Can you work these out from the model? Positions are in its coordinate system, mm. A direction names the side the tool comes from. Coordinates: 2 decimals unless noted, no trailing zeros. Order: outer loops, then holes, each group sorted by start corner. A loop starts at its lowest first (then second) coordinate and runs counter-clockwise, first axis right, second up. Notation, with made-up numbers: M -30,33 L 14,33 A14 ccw 14,44 Z; hole C 35.25,5.25 d8. An arc over 180 degrees is marked long. Answer as a JSON object with one key per item and string values.
from build123d import *

# Parameters (mm, degrees)
F1_DEPTH = 5.9944
F0_R     = 5.9944
F2_DEPTH = 13.0048
F0_R_2   = 13.0048
F3_DEPTH = 20.0025


with BuildPart() as f1:
    # F0 (on Front) → F1 (new body)
    with BuildSketch(Plane.XZ):
        with BuildLine():
            ThreePointArc((-12.0015, 0), (0, 12.0015), (12.0015, 0))
            ThreePointArc((12.0015, 0), (10.942664, -4.928905), (7.952988, -8.988102))
            Line((7.952988, -8.988102), (71.316989, 47.078591))
            ThreePointArc((71.316989, 47.078591), (78.103737, 50.03276), (85.331821, 48.438437))
            ThreePointArc((85.331821, 48.438437), (73.022425, 71.33485), (87.698507, 92.791308))
            Line((87.698507, 92.791308), (-4.940825, 50.942287))
            ThreePointArc((-4.940825, 50.942287), (6.509174, 50.087989), (12.0015, 40.005))
            ThreePointArc((12.0015, 40.005), (0, 28.0035), (-12.0015, 40.005))
            Line((-12.0015, 40.005), (-12.0015, 0))
        make_face()
    extrude(amount=F1_DEPTH)

    # F0 (on Front) → F2 (join)
    with BuildSketch(Plane.XZ):
        with BuildLine():
            ThreePointArc((-4.940825, 50.942287), (-10.082989, 46.514174), (-12.0015, 40.005))
            ThreePointArc((-12.0015, 40.005), (0, 28.0035), (12.0015, 40.005))
            ThreePointArc((12.0015, 40.005), (6.509174, 50.087989), (-4.940825, 50.942287))
        make_face()
        with Locations((0, 40.005)):
            Circle(F0_R, mode=Mode.SUBTRACT)
        with BuildLine():
            ThreePointArc((7.952988, -8.988102), (10.942664, -4.928905), (12.0015, 0))
            ThreePointArc((12.0015, 0), (0, 12.0015), (-12.0015, 0))
            ThreePointArc((-12.0015, 0), (-4.928905, -10.942664), (7.952988, -8.988102))
        make_face()
        Circle(F0_R, mode=Mode.SUBTRACT)
    extrude(amount=F2_DEPTH)

    # F0 (on Front) → F3 (join)
    with BuildSketch(Plane.XZ):
        with BuildLine():
            ThreePointArc((87.698507, 92.791308), (73.022425, 71.33485), (85.331821, 48.438437))
            ThreePointArc((85.331821, 48.438437), (110.416984, 48.30068), (122.9995, 70.0024))
            ThreePointArc((122.9995, 70.0024), (111.555701, 91.011294), (87.698507, 92.791308))
        make_face()
        with Locations((97.9932, 70.0024)):
            Circle(F0_R_2, mode=Mode.SUBTRACT)
    extrude(amount=F3_DEPTH)

    # F4: F1 across plane


with BuildPart() as f1_1:
    add(f1.part)
    add(f1.part.mirror(Plane.XZ))


solid = f1_1.part
Item 1: I want a section at C-C, the plane x = 96. Write out the boundary of the cut face in (y, z), plus the area to 3 significant figures.
Answers follow:
{"outline": "M -20,45.08 L 20,45.08 L 20,57.15 L -20,57.15 Z; M -20,82.85 L 20,82.85 L 20,94.93 L -20,94.93 Z", "area": "966 mm^2"}
Item 2: I want a section at A-A, the plane y = 8. Write out the boundary of the cut face in (x, z) (1 decimal), plus the area to 3 significant figures.
Answers follow:
{"outline": "C 0,0 d24; M -12,40 A12 ccw long -4.9,50.9 A12 ccw Z; M 85.3,48.4 A25 ccw 123,70 A25 ccw long Z; hole C 0,0 d12; hole C 0,40 d12; hole C 98,70 d26", "area": "2,110 mm^2"}
Item 3: Which directions (+Z, -Z, +X, -X, +Y, -Y) give clear straight access to the entire face, cutting with the end or side of a thin tool? Please do faces 5 (the flat face through (-6, -13.005, 38)), 6 (the flat face through (42.03, -0.08, 72.16)), 7 (the flat face through (-6, 13.005, 38)).
Answers follow:
{"face 5": "+Z, -Z, -X, -Y", "face 6": "+Z, -X, +Y, -Y", "face 7": "+Z, -Z, -X, +Y"}
Item 4: I want a section at B-B, the plane x = 0. Write out the boundary of the cut face in (y, z), plus the area to 3 significant figures.
Answers follow:
{"outline": "M -13,-12 L 13,-12 L 13,-5.99 L -13,-5.99 Z; M -13,5.99 L 13,5.99 L 13,12 L 5.99,12 L 5.99,28 L 13,28 L 13,34.01 L -13,34.01 L -13,28 L -5.99,28 L -5.99,12 L -13,12 Z; M -13,46 L 13,46 L 13,52.01 L 5.99,52.01 L 5.99,53.17 L -5.99,53.17 L -5.99,52.01 L -13,52.01 Z", "area": "831 mm^2"}
Item 5: If we mould it in two halves opening along Z, with no side actions, what happens to faces 1 (the cylindrical face through (110.006, 0.28, 65.021)), 2 (the flat face through (2, -13.005, 6)), 3 (the cylindrical face through (77.999, -0.084, 50.022)), 4 (the cylindrical face through (5.718, 0.182, 1.801))? For each: pulls with the +Z half, pulls with the -Z half, needs draft (parallel to the pull), parting line crosses it, or undercut.
Answers follow:
{"face 1": "undercut", "face 2": "needs draft", "face 3": "pulls with the -Z half", "face 4": "undercut"}
Item 6: Please list where these lines run through material, in increasing order: line 1 (Z direction, x = -2.5, y = -7.5); line 2 (Z direction, x = 0, y = -1.25); line 3 (X direction, y = 18.5, z = 59).
Answers follow:
{"line 1": "z = -11.74 to -5.45, 5.45 to 11.74, 28.27 to 34.56, 45.45 to 51.74", "line 2": "z = -12 to -5.99, 5.99 to 34.01, 46 to 53.17", "line 3": "x = 75.54 to 91.06, 104.93 to 120.45"}
Item 7: I'm going to push flat-ended pins straight in: pin 1 (19 mm diameter, centred on x = -4, z = 41.5, fed in from +Y); pin 2 (1.5 mm diameter, centred on y = 0.5, z = 29.5, fed in from +X); pin 3 (7 mm diameter, centred on x = 0, z = 0, fed in from +Y); pin 4 (6 mm diameter, centred on x = 79.5, y = 8.5, fed in from +Z). Where does each tip first touch, or does it pass through?
Answers follow:
{"pin 1": "stops at y = 13", "pin 2": "stops at x = 52.3", "pin 3": "passes through", "pin 4": "stops at z = 89.83"}
Item 8: I want a section at D-D, the plane y = -2. Write out the boundary of the cut face in (x, z) (1 decimal).
Answers follow:
{"outline": "M -12,0 A12 ccw 8,-9 L 71.3,47.1 A12 cw 85.3,48.4 A25 ccw 123,70 A25 ccw 87.7,92.8 L -4.9,50.9 A12 ccw -12,40 Z; hole C 0,0 d12; hole C 0,40 d12; hole C 98,70 d26"}
